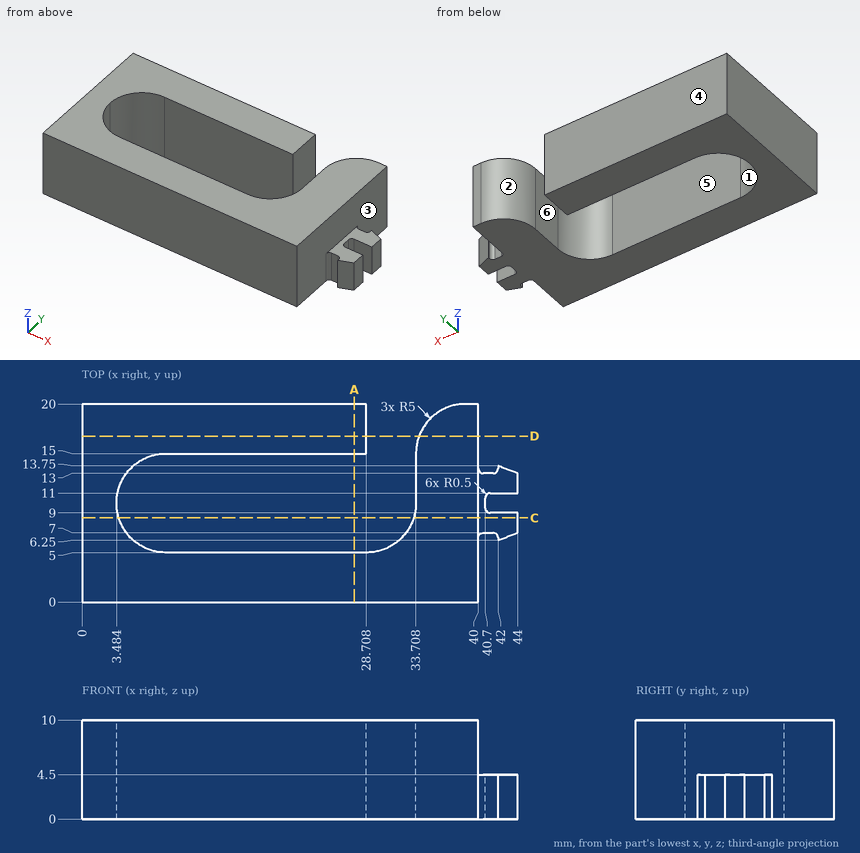
Could you check a few things on this drawing? It's one solid part, dimensions in mm from its lowest x, y, z. A direction names the side the tool comes from. Round coordinates to 2 decimals unless told otherwise and drop trailing zeros. Write each loop counter-clockwise with the first axis right and the second up, starting at its lowest first coordinate (ties: lowest second). Pieces come first, ordered by that corner, then holes. Notation, with made-up numbers: (36, -12.5) -> (77, -12.5) arc R21 ccw to (77, -2.5) -> close; hole circle Ø5 at (39.25, -24). An arc over 180 degrees is marked (long way). Use one line per item in the form item = value. Start each with the question number.
Q1. If I drill on probe 1 along Y at (x, z) = (28.5, 1.5); probe 2 along X at (y, z) = (15.25, 8.75) (1 decimal); probe 3 along X at (y, z) = (8.5, 6.5) (1 decimal), over which ranges is the centre line in solid material (lowest first)? Write a range as [from, to].
Q2. Imagine slicing it at D-D (y = 16.75). Please give me the cut outline in (x, z), then the cut area to 3 significant figures.
Q3. I'm going to push flat-ended pins straight in: P1, Ø1.4, axis at x = 42.5, z = 2.5, coming from the -Y side; P2, Ø3, axis at x = 43, z = 1.5, coming from the +Y side; P3, Ø1.1, axis at x = 41, z = 2.5, coming from the -Y side. Where does each tip first touch, or does it pass through?
Q4. Imagine slicing it at C-C (y = 8.5). Please give me the cut outline in (x, z).
Q5. We'd pull the mould along Y, two halves only. Please class the marked faces 1, 2 and 3: +Y half, -Y half, draft (parallel to the pull), parting line (faces both ways), or undercut.
Q6. Which directions (+Z, -Z, +X, -X, +Y, -Y) give clear straight access to the entire face, cutting with the end or side of a thin tool? Please do the marked faces 4, 5 and 6.
Q7. Imagine slicing it at A-A (x = 27.5). Please give me the cut outline in (y, z), then the cut area to 3 significant figures.
Worked out:
q1.probe_1 = [0, 5], [15, 20]
q1.probe_2 = [0, 28.7], [33.7, 40]
q1.probe_3 = [0, 3.7], [33.5, 40]
q2.outline = (0, 0) -> (28.71, 0) -> (28.71, 10) -> (0, 10) -> close; (34.02, 0) -> (40, 0) -> (40, 10) -> (34.02, 10) -> close
q2.area = 347 mm^2
q3.P1 = 6.25
q3.P2 = 13.75
q3.P3 = 7
q4.outline = (0, 0) -> (3.71, 0) -> (3.71, 10) -> (0, 10) -> close; (33.48, 0) -> (44, 0) -> (44, 4.5) -> (40, 4.5) -> (40, 10) -> (33.48, 10) -> close
q5.face_1 = undercut
q5.face_2 = +Y half
q5.face_3 = draft
q6.face_4 = +Z, -Z, +X, -X, +Y
q6.face_5 = +Z, -Z
q6.face_6 = +Z, -Z, +Y
q7.outline = (0, 0) -> (5, 0) -> (5, 10) -> (0, 10) -> close; (15, 0) -> (20, 0) -> (20, 10) -> (15, 10) -> close
q7.area = 100 mm^2
